The model under review builds one solid part; all positions refer to its coordinate system, in mm. A direction names the side the tool comes from. Coordinates: 2 decimals unless noted, no trailing zeros. Write each loop counter-clockwise with the first axis right and the second up, starting at its lowest first coordinate (ties: lowest second). Pieces come first, ordered by that corner, then holes. Notation, with made-up numbers: (30.5, -21.75) - (67.5, -21.75) arc R27 cw to (67.5, 5.25) - close; hole circle Ø1 at (73.5, -0.5). An arc over 180 degrees is marked (long way). Return JSON: item names as keys, results as strings. Group by question number.
(1) Tool access review of faces 1 (the face through (60, 37, 15)), 2 (the face through (47, 29, 19)), 3 (the face through (82, 5, 24)), 4 (the face through (71, 18, 19)): name each direction out of +Z, -Z, +X, -X, +Y, -Y from which nothing blocks a thin tool from reaching the whole face with its end or side.
(2) We need section A-A on z = 16. State the section outline as (x, y) points.
(3) Draft analysis for pull direction Z (two halves, no side actions). For faces 5 (the face through (48, 18, 0)), 6 (the face through (94, 9, 5)), 7 (the face through (8, 13, 28)), 8 (the face through (12, 5, 24)), state which applies: released by +Z, released by -Z, zero draft, split by the parting line, or undercut.
(4) We need section D-D on z = 33. State the section outline as (x, y) points, then the cut area to 3 significant figures.
(5) We need section B-B on y = 34.5. State the section outline as (x, z) points, then the cut area to 3 significant figures.
(6) We need section C-C on x = 60. State the section outline as (y, z) points, then the cut area to 3 significant figures.
(7) To check wall thickness, follow L1, parallel to Z at x = 9, y = 6.5; L2, parallel to Z at x = 4.5, y = 11; L3, parallel to Y at x = 72, z = 23.5. State the ranges of each line that lie inside material, in increasing order. Write a range as from..to.
(8) For pin 1 Ø4 at (y, z) = (31.5, 33.5) entering from -X; pin 2 Ø3.5 at (y, z) = (3, 21.5) entering from -X; pin 3 Ø1.5 at (x, z) = (64, 19) entering from +Y, all flat-tipped, find the tip position at first contact; note any pin that passes through.
```python
from build123d import *

# Parameters (mm, degrees)
BOSS_EXTRUDE1_DEPTH = 38
CUT_EXTRUDE1_DEPTH  = 16
SKETCH4_W           = 28.425340807
SKETCH4_H           = 18
CUT_EXTRUDE2_DEPTH  = 46
SKETCH5_W           = 11.74
SKETCH5_H           = 10
CUT_EXTRUDE3_DEPTH  = 76


with BuildPart() as part:
    # Sketch1 → Boss-Extrude1 (new body)
    with BuildSketch(Plane.XY):
        Polygon((0, 0), (0, 18), (31, 18), (31, 45), (63, 45), (63, 18), (94, 18), (94, 0), align=None)
    extrude(amount=BOSS_EXTRUDE1_DEPTH)

    # Sketch2 → Cut-Extrude1 (cut)
    with BuildSketch(Plane(origin=(0, 45, 0), x_dir=(1, 0, 0), z_dir=(0, 1, 0))):
        with BuildLine():
            Line((63, -23), (63, -15))
            Line((63, -15), (56.16515139, -15))
            ThreePointArc((56.16515139, -15), (47, -9), (37.83484861, -15))
            Line((37.83484861, -15), (31, -15))
            Line((31, -15), (31, -23))
            Line((31, -23), (37.83484861, -23))
            ThreePointArc((37.83484861, -23), (47, -29), (56.16515139, -23))
            Line((56.16515139, -23), (63, -23))
        make_face()
    extrude(amount=-CUT_EXTRUDE1_DEPTH, mode=Mode.SUBTRACT)

    # Sketch4 → Cut-Extrude2 (cut)
    with BuildSketch(Plane(origin=(0, 0, 0), x_dir=(-0.773957299203321, -0.6332377902572627, 0), z_dir=(0.6332377902572627, -0.773957299203321, 0))):
        with Locations((-14.212670404, -19)):
            Rectangle(SKETCH4_W, SKETCH4_H)
    cut_extrude2 = extrude(amount=-CUT_EXTRUDE2_DEPTH, mode=Mode.SUBTRACT)

    # Sketch5 → Cut-Extrude3 (cut)
    with BuildSketch(Plane(origin=(0, 18, 0), x_dir=(1, 0, 0), z_dir=(0, 1, 0))):
        with Locations((11, -19)):
            Rectangle(SKETCH5_W, SKETCH5_H)
    cut_extrude3 = extrude(amount=-CUT_EXTRUDE3_DEPTH, mode=Mode.SUBTRACT)

    # Mirror1: Cut-Extrude2, Cut-Extrude3 across plane
    add(cut_extrude2.mirror(Plane(origin=(47, 0, 0), x_dir=(0, 0, 1), z_dir=(1, 0, 0))), mode=Mode.SUBTRACT)
    add(cut_extrude3.mirror(Plane(origin=(47, 0, 0), x_dir=(0, 0, 1), z_dir=(1, 0, 0))), mode=Mode.SUBTRACT)


solid = part.part
```
Ans:
{
 "1": {"face 1": "+X, -X, +Y", "face 2": "+Y", "face 3": "+Y, -Y", "face 4": "+Z, -Z, +X, +Y"},
 "2": {"outline": "(0, 0) - (5.13, 0) - (5.13, 4.2) - close; (16.87, 0) - (77.13, 0) - (77.13, 13.8) - (72, 18) - (63, 18) - (63, 29) - (31, 29) - (31, 18) - (22, 18) - (16.87, 13.8) - close; (88.87, 0) - (94, 0) - (88.87, 4.2) - close"},
 "3": {"face 5": "released by -Z", "face 6": "zero draft", "face 7": "undercut", "face 8": "undercut"},
 "4": {"outline": "(0, 0) - (94, 0) - (94, 18) - (63, 18) - (63, 45) - (31, 45) - (31, 18) - (0, 18) - close", "area": "2,560 mm²"},
 "5": {"outline": "(31, 0) - (63, 0) - (63, 15) - (56.17, 15) arc R10 cw to (37.83, 15) - (31, 15) - close; (31, 23) - (37.83, 23) arc R10 cw to (56.17, 23) - (63, 23) - (63, 38) - (31, 38) - close", "area": "801 mm²"},
 "6": {"outline": "(0, 0) - (45, 0) - (45, 15) - (29, 15) - (29, 23) - (45, 23) - (45, 38) - (0, 38) - close", "area": "1,580 mm²"},
 "7": {"L1": "0..14, 24..38", "L2": "0..10, 28..38", "L3": "0..18"},
 "8": {"pin 1": "x = 31", "pin 2": "x = 1.53", "pin 3": "y = 18"}
}
